Can you work these out from the model? Positions are in its coordinate system, mm. Face numbers are marked on the shaded views. A direction names the side the tool comes from. Give positions to 0.01 mm unless a question says otherwise; leave off trailing zeros. Loops run counter-clockwise (first coordinate to the right, second up) from the corner with the lowest first, then second, coordinate; pieces in that order, holes last. Notation, with made-up numbers: (56.5, 53) -> (111.5, 53) arc R17 ccw to (111.5, 83) -> close; hole circle Ø7 at (80.5, 9). An arc over 180 degrees is marked (long way). One line per question, with ' | ' between items.
from build123d import *

# Parameters (mm, degrees)
SKETCH1_W           = 38
SKETCH1_H           = 12
BOSS_EXTRUDE1_DEPTH = 15
SKETCH2_R           = 1.15
CUT_EXTRUDE1_DEPTH  = 15
SKETCH3_W           = 20
SKETCH3_H           = 15
CUT_EXTRUDE2_DEPTH  = 5
CUT_EXTRUDE3_START  = -6
SKETCH2_3_R         = 2.5
CUT_EXTRUDE3_DEPTH  = 9
SKETCH4_W           = 23.485116632
SKETCH4_H           = 8.604460082
CUT_EXTRUDE4_DEPTH  = 5
SKETCH5_R           = 3.886662334
CUT_EXTRUDE5_DEPTH  = 2


with BuildPart() as part:
    # Sketch1 → Boss-Extrude1 (new body)
    with BuildSketch(Plane(origin=(0, 0, 0), x_dir=(1, 0, 0), z_dir=(0, 1, 0))):
        with Locations((19, 6)):
            Rectangle(SKETCH1_W, SKETCH1_H)
    extrude(amount=BOSS_EXTRUDE1_DEPTH)

    # Sketch2 → Cut-Extrude1 (cut)
    with BuildSketch(Plane.ZY):
        with Locations((-3, 11)):
            Circle(SKETCH2_R)
    extrude(amount=-CUT_EXTRUDE1_DEPTH, mode=Mode.SUBTRACT)

    # Sketch3 → Cut-Extrude2 (cut)
    with BuildSketch(Plane.XY):
        with Locations((25, 7.5)):
            Rectangle(SKETCH3_W, SKETCH3_H)
    extrude(amount=-CUT_EXTRUDE2_DEPTH, mode=Mode.SUBTRACT)

    # Sketch2<3> → Cut-Extrude3 (cut)
    with BuildSketch(Plane.ZY.offset(CUT_EXTRUDE3_START)):
        with Locations((-3, 11)):
            Circle(SKETCH2_3_R)
    extrude(amount=-CUT_EXTRUDE3_DEPTH, mode=Mode.SUBTRACT)

    # Sketch4 → Cut-Extrude4 (cut)
    with BuildSketch(Plane(origin=(0, 0, -12), x_dir=(-1, 0, 0), z_dir=(0, 0, -1))):
        with Locations((-21.50003141, 4.302230041)):
            Rectangle(SKETCH4_W, SKETCH4_H)
    extrude(amount=-CUT_EXTRUDE4_DEPTH, mode=Mode.SUBTRACT)

    # Sketch5 → Cut-Extrude5 (cut)
    with BuildSketch(Plane.XY.offset(-5)):
        with Locations((30.325082157, 3.904217079)):
            Circle(SKETCH5_R)
    extrude(amount=-CUT_EXTRUDE5_DEPTH, mode=Mode.SUBTRACT)


solid = part.part
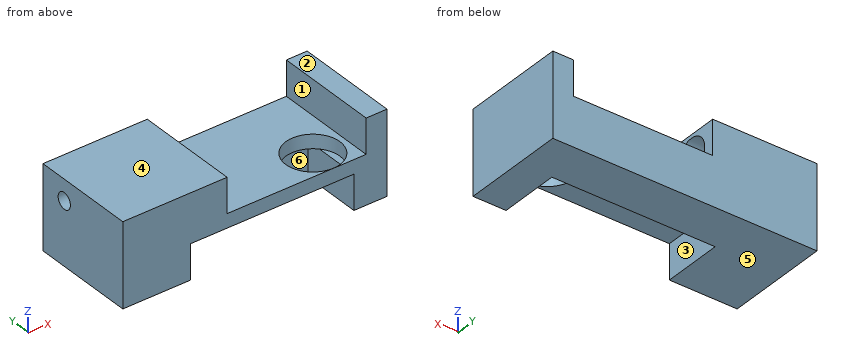
Q1. If we section it at C-C (x = 6.5): Write out the boundary of the cut face in (y, z), plus the area to 3 significant figures.
Entries:
outline: (0, -12) -> (15, -12) -> (15, 0) -> (0, 0) -> close; hole circle Ø5 at (11, -3) | area: 160 mm²
Q2. If we section it at A-A (z = -1.5): Write out the boundary of the cut face in (x, y), plus the area to 3 significant figures.
Entries:
outline: (0, 0) -> (15, 0) -> (15, 9) -> (6, 9) -> (6, 13) -> (15, 13) -> (15, 15) -> (0, 15) -> close; (35, 0) -> (38, 0) -> (38, 15) -> (35, 15) -> close | area: 234 mm²
Q3. If we section it at D-D (z = -3): Write out the boundary of the cut face in (x, y).
Entries:
outline: (0, 0) -> (15, 0) -> (15, 8.5) -> (6, 8.5) -> (6, 9.85) -> (0, 9.85) -> close; (0, 12.15) -> (6, 12.15) -> (6, 13.5) -> (15, 13.5) -> (15, 15) -> (0, 15) -> close; (35, 0) -> (38, 0) -> (38, 15) -> (35, 15) -> close
Q4. If I drill on probe 1 along X at (y, z) = (7.5, -8.5); probe 2 along X at (y, z) = (12.75, -3.75); probe 3 along Y at (x, z) = (7, -5), over which ranges is the centre line in solid material (lowest first)? Write a range as from..to.
Entries:
probe 1: 0..9.76, 33.24..38 | probe 2: 0..6, 35..38 | probe 3: 0..9.5, 12.5..15
Q5. For pin 1 Ø4.5 at (y, z) = (11, -3) entering from -X; pin 2 Ø2 at (x, y) = (31.5, 7.5) entering from -Z; pin 3 Ø3 at (x, y) = (17, 10.5) entering from +Z; pin 4 Ø1.1 at (x, y) = (33.5, 4.5) entering from +Z, each with a flat end and sliding along its axis, tell me the tip position at first contact or that it passes through.
Entries:
pin 1: x = 0 | pin 2: z = -7 | pin 3: z = -5 | pin 4: z = -7
Q6. On a 3-axis mill with a long thin cutter (end or side, diameter ignored), from which of +Z, -Z, +X, -X, +Y, -Y can I reach the whole of each face in a straight line? I mean the marked faces 1, 2 and 3. Say none if no direction works.
Entries:
face 1: +Z, +Y, -Y | face 2: +Z, +X, -X, +Y, -Y | face 3: -Z, -Y
Q7. If we section it at B-B (y = 11): Write out the boundary of the cut face in (x, z), plus the area to 3 significant figures.
Entries:
outline: (0, -12) -> (38, -12) -> (38, 0) -> (35, 0) -> (35, -5) -> (15, -5) -> (15, -5.5) -> (6, -5.5) -> (6, -4.15) -> (0, -4.15) -> close; (0, -1.85) -> (6, -1.85) -> (6, -0.5) -> (15, -0.5) -> (15, 0) -> (0, 0) -> close | area: 297 mm²
Q8. If we mould it in two halves opening along Z, with no side actions, what happens to the marked faces 4, 5 and 6? For each: pulls with the +Z half, pulls with the -Z half, needs draft (parallel to the pull), parting line crosses it, or undercut.
Entries:
face 4: pulls with the +Z half | face 5: pulls with the -Z half | face 6: needs draft
